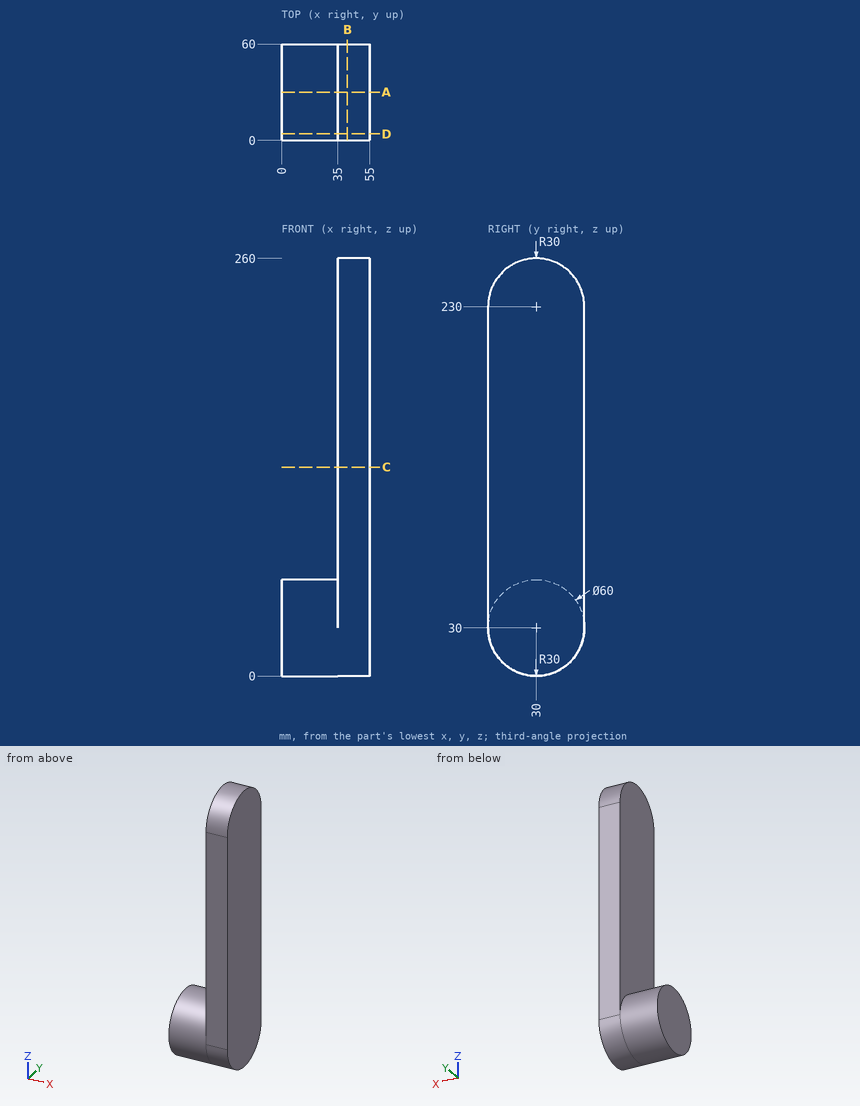
Print and shaded views of the part. All mm, measured from the part's lowest x, y and z. Coordinates: 2 decimals unless noted, no trailing zeros. Loops run counter-clockwise (first coordinate to the right, second up) from the corner with the lowest first, then second, coordinate; pieces in that order, holes last. Notation, with made-up numbers: M 46.25,87.5 L 84.25,87.5 A9 ccw 84.25,95.5 Z; hole C 43.25,-30.75 d10. An arc over 180 degrees is marked long. Use a Markdown table: item, result. Add a question column.
Q1. Probe L1, parallel to Y at x = 22, z = 31.5; L2, parallel to X at y = 54, z = 206.5; L3, parallel to Z at x = 23, y = 55. List the from-to ranges inside material, lowest first.
Q2. Pin check, flat tips, straight feed: P1, Ø5, axis at x = 25, y = 42, coming from the +Z side; P2, Ø18, axis at y = 40, z = 150, coming from the -X side. Stop position of each tip, or through.
Q3. Cut at C-C (z = 130). Write the cut outline in (x, y), and give its area (3 significant figures).
Q4. Cut at A-A (y = 30). Write the cut outline in (x, z).
Q5. Cut at D-D (y = 4). Write the cut outline in (x, z), and give its area (3 significant figures).
Q6. Cut at B-B (x = 41). Write the cut outline in (y, z).
Worked out:
| question | item | result |
|---|---|---|
| 1 | L1 | y = 0.04 to 59.96 |
| 1 | L2 | x = 35 to 55 |
| 1 | L3 | z = 13.42 to 46.58 |
| 2 | P1 | stops at z = 58.46 |
| 2 | P2 | stops at x = 35 |
| 3 | outline | M 35,0 L 55,0 L 55,60 L 35,60 Z |
| 3 | area | 1,200 mm2 |
| 4 | outline | M 0,0 L 55,0 L 55,260 L 35,260 L 35,60 L 0,60 Z |
| 5 | outline | M 0,15.03 L 55,15.03 L 55,244.97 L 35,244.97 L 35,44.97 L 0,44.97 Z |
| 5 | area | 5,650 mm2 |
| 6 | outline | M 0,30 A30 ccw 60,30 L 60,230 A30 ccw 0,230 Z |
